```python
from build123d import *

# Parameters (mm, degrees)
F1_R     = 19.05
F3_DEPTH = 3.175


with BuildPart() as f2:
    # F1 (on Right) → F2 (revolve)
    with BuildSketch(Plane.YZ):
        with Locations((0, 177.8004914522)):
            Circle(F1_R)
    revolve(axis=Axis((0, 0, 0), (0, -1, 0)))

    # F0 (on Front) → F3 (join, symmetric)
    with BuildSketch(Plane.XZ):
        with BuildLine():
            Line((-19.05, -19.05), (-19.05, 19.05))
            Line((-19.05, 19.05), (-177.3458485559, 12.7))
            Line((-177.3458485559, 12.7), (-165.1, 12.7))
            Line((-165.1, 12.7), (-165.1, -12.7))
            Line((-165.1, -12.7), (-177.3458485559, -12.7))
            ThreePointArc((-177.3458485559, -12.7), (-177.3451960004, -12.7091091572), (-177.3445429771, -12.7182182809))
            Line((-177.3445429771, -12.7182182809), (-19.05, -19.05))
        make_face()
        with BuildLine():
            Line((165.1, 12.7), (177.3458485559, 12.7))
            Line((177.3458485559, 12.7), (19.05, 19.05))
            Line((19.05, 19.05), (12.7182182809, 177.3445429771))
            ThreePointArc((12.7182182809, 177.3445429771), (12.7091091572, 177.3451960004), (12.7, 177.3458485559))
            Line((12.7, 177.3458485559), (12.7, 165.1))
            Line((12.7, 165.1), (-12.7, 165.1))
            Line((-12.7, 165.1), (-12.7, 177.3458485559))
            ThreePointArc((-12.7, 177.3458485559), (-12.7091091572, 177.3451960004), (-12.7182182809, 177.3445429771))
            Line((-12.7182182809, 177.3445429771), (-19.05, 19.05))
            Line((-19.05, 19.05), (-19.05, -19.05))
            Line((-19.05, -19.05), (-12.7, -177.3458485559))
            Line((-12.7, -177.3458485559), (-12.7, -165.1))
            Line((-12.7, -165.1), (12.7, -165.1))
            Line((12.7, -165.1), (12.7, -177.3458485559))
            ThreePointArc((12.7, -177.3458485559), (12.7091091572, -177.3451960004), (12.7182182809, -177.3445429771))
            Line((12.7182182809, -177.3445429771), (19.05, -19.05))
            Line((19.05, -19.05), (177.3445429771, -12.7182182809))
            ThreePointArc((177.3445429771, -12.7182182809), (177.3451960004, -12.7091091572), (177.3458485559, -12.7))
            Line((177.3458485559, -12.7), (165.1, -12.7))
            Line((165.1, -12.7), (165.1, 12.7))
        make_face()
    extrude(amount=F3_DEPTH, both=True)


solid = f2.part
```
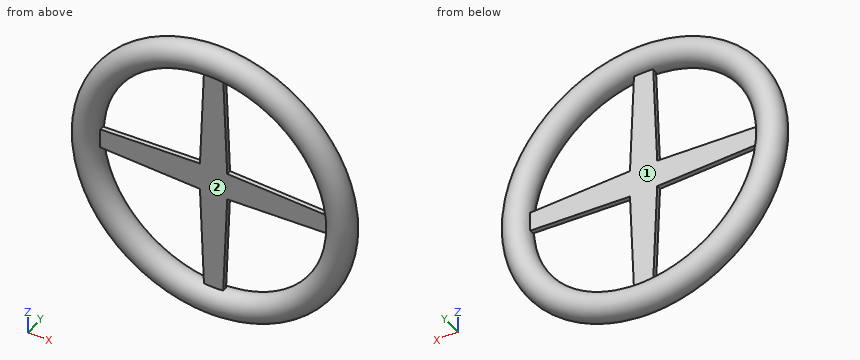
The listing builds one solid part. Answer for the finished solid, in the listing's coordinates (mm). Face numbers are marked on the shaded views. Coordinates: 2 decimals unless noted, no trailing zeros. Loops run counter-clockwise (first coordinate to the right, second up) from the corner with the lowest first, then second, coordinate; pieces in that order, holes last. Notation, with made-up numbers: (61.5, 6.5) -> (72.5, 6.5) arc R19 ccw to (72.5, 21.5) -> close; hole circle Ø2 at (64.25, -21.5). An arc over 180 degrees is marked (long way). Return JSON: item names as keys, results as strings. Group by question number.
(1) A cutting plane is placed at B-B on x = 111.5. Count the separate pieces of the cut face and the enclosed holes in it, and give its area (3 significant figures).
(2) Find the intervals of material crossed by probe 1 along X at (y, z) = (-7.5, 35.5); probe 2 along X at (y, z) = (0, -78.5); probe 3 along X at (y, z) = (-12.5, -70), in increasing order. Write a range as from..to.
(3) A cutting plane is placed at A-A on y = 9.5. Write down the section's boundary in (x, z).
(4) Given pin 1 Ø10 at (x, z) = (155.5, 125.5) entering from +Y; pin 2 Ø12 at (y, z) = (4, 108.5) entering from +X; pin 3 Ø12 at (y, z) = (-9, 97.5) entering from -X; pin 4 Ø10 at (x, z) = (-124, 23.5) entering from +Y (3 decimals), each flat-ended and moving along its own axis, determine where each tip first touches the part or whether it passes through.
(5) Determine the mould class of the marked faces 1 and 2 for opening direction X: released by +X, released by -X, zero draft, split by the parting line, or undercut.
The answers:
{
 "1": {"separate pieces": "3", "enclosed holes": "0", "area": "3,140 mm^2"},
 "2": {"probe 1": "x = -192.06..-156.31, 156.31..192.06", "probe 2": "x = -180.52..-137.98, -16.67..16.67, 137.98..180.52", "probe 3": "x = -178.97..-147.67, 147.67..178.97"},
 "3": {"outline": "circle Ø388.63 at (0, 0); hole circle Ø322.58 at (0, 0)"},
 "4": {"pin 1": "stops at y = 8.55", "pin 2": "stops at x = 167.75", "pin 3": "stops at x = -172.78", "pin 4": "passes through"},
 "5": {"face 1": "undercut", "face 2": "undercut"}
}
